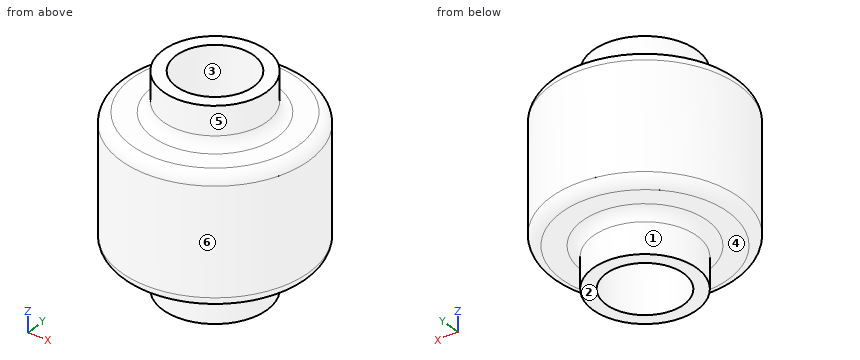
```python
from build123d import *

# Parameters (mm, degrees)
F0_R       = 45.4520962522
F1_DEPTH   = 61.59209
F2_R       = 25.1143263765
F1_FACE1_R = 45.4520962522
F3_DEPTH   = 18.93017
F4_R       = 25.1788729995
F5_DEPTH   = 19.9562
F6_R       = 5.08
F7_R       = 18.7687787906
F8_DEPTH   = 284.89901


with BuildPart() as f1:
    # F0 (on Top) → F1 (new body)
    with BuildSketch(Plane.XY):
        Circle(F0_R)
    extrude(amount=F1_DEPTH)

    # F2 (on face) + F1_face1 (on face) → F3 (join)
    with BuildSketch(Plane.XY.offset(61.59209)):
        Circle(F2_R)
    with BuildSketch(Plane(origin=(0, 0, 0), x_dir=(1, 0, 0), z_dir=(0, 0, -1))):
        Circle(F1_FACE1_R)
    extrude(amount=F3_DEPTH, dir=(0, 0, 1))

    # F4 (on face) → F5 (join)
    with BuildSketch(Plane(origin=(0, 0, 0), x_dir=(1, 0, 0), z_dir=(0, 0, -1))):
        Circle(F4_R)
    extrude(amount=F5_DEPTH)

    # F6
    f6_edges = [f1.edges().sort_by_distance(p)[0] for p in [
        (-45.452096, 0, 0),
        (45.452096, 0, 30.796045),
        (-45.452096, 0, 61.59209),
        (-25.114326, 0, 61.59209),
        (-25.178873, 0, 0),
    ]]
    fillet(f6_edges, radius=F6_R)

    # F7 (on face) → F8 (cut)
    with BuildSketch(Plane.XY.offset(80.52226)):
        Circle(F7_R)
    extrude(amount=-F8_DEPTH, mode=Mode.SUBTRACT)


solid = f1.part
```
For this review, take the finished solid that the model builds, in its own axes (mm). Face numbers are marked on the shaded views. A direction names the side the tool comes from. Round coordinates to 2 decimals unless told otherwise and drop trailing zeros. Order: outer loops, then holes, each group sorted by start corner. A loop starts at its lowest first (then second) coordinate and runs counter-clockwise, first axis right, second up.
Q1. We need section C-C, the plane z = 21. Give the boundary of the cut face in (x, y), plus the area to 3 significant figures.
Findings below:
outline: circle Ø90.9 at (0, 0); hole circle Ø37.54 at (0, 0)
area: 5,380 mm2
Q2. Mouldability with a two-part tool opening along X and no side actions: class the marked faces 1, 2 and 3 as pulls with the +X half, pulls with the -X half, needs draft (parallel to the pull), parting line crosses it, or undercut.
Findings below:
face 1: parting line crosses it
face 2: needs draft
face 3: undercut
Q3. Machinability: for the marked faces 4, 5 and 6, which of the approach directions +Z, -Z, +X, -X, +Y, -Y give a long, thin tool a straight path to every point of the face, cutting with its end or side? Answer none if there is none.
Findings below:
face 4: -Z
face 5: +Z
face 6: +Z, -Z
Q4. Insertion check: P1, Ø6, axis at y = 4.5, z = 68.5, coming from the +X side; P2, Ø6, axis at y = -34.5, z = 34, coming from the -X side; P3, Ø3, axis at x = -27.5, z = 4, coming from the -Y side. Each pin has a flat end and moves straight along its axis. Give the tip position at first contact, or say it passes through.
Findings below:
P1: stops at x = 25.07
P2: stops at x = -32.77
P3: stops at y = -37.19
Q5. We need section A-A, the plane y = 0. Give the boundary of the cut face in (x, z).
Findings below:
outline: (-45.45, 5.08) arc R5.08 ccw to (-40.37, 0) - (-30.26, 0) arc R5.08 cw to (-25.18, -5.08) - (-25.18, -19.96) - (-18.77, -19.96) - (-18.77, 80.52) - (-25.11, 80.52) - (-25.11, 66.67) arc R5.08 cw to (-30.19, 61.59) - (-40.37, 61.59) arc R5.08 ccw to (-45.45, 56.51) - close; (18.77, -19.96) - (25.18, -19.96) - (25.18, -5.08) arc R5.08 cw to (30.26, 0) - (40.37, 0) arc R5.08 ccw to (45.45, 5.08) - (45.45, 56.51) arc R5.08 ccw to (40.37, 61.59) - (30.19, 61.59) arc R5.08 cw to (25.11, 66.67) - (25.11, 80.52) - (18.77, 80.52) - close
Q6. Wall thickness on line 1 (Y direction, x = 0, z = 51.5); line 2 (X direction, y = -11, z = 27); line 3 (Z direction, x = 35, y = 0): over which ranges is each line inside the solid? List them lowest first.
Findings below:
line 1: y = -45.45 to -18.77, 18.77 to 45.45
line 2: x = -44.1 to -15.21, 15.21 to 44.1
line 3: z = 0 to 61.59
